For this review, take the finished solid that the model builds, in its own axes (mm). A direction names the side the tool comes from. Coordinates: 2 decimals unless noted, no trailing zeros. Loops run counter-clockwise (first coordinate to the right, second up) from the corner with the lowest first, then second, coordinate; pieces in that order, holes last. Notation, with made-up numbers: (47, 88) - (73, 88) arc R9 ccw to (73, 93) - close; hole circle Ø7 at (30.25, 54). An arc over 180 degrees is marked (long way). Use one line per item in the form item = value. Start each with the question number.
1. Machinability: for faces 1 (the face through (-0.33, -2.52, 3.76)), 2 (the face through (0, 0, -66.548)), which of the approach directions +Z, -Z, +X, -X, +Y, -Y give a long, thin tool a straight path to every point of the face, cutting with its end or side? Answer none if there is none.
2. For pin 1 Ø3 at (x, z) = (15.5, -5) entering from +Y; pin 2 Ø10 at (y, z) = (-14.5, -8.5) entering from +X; pin 3 Ø5 at (y, z) = (14.5, -31.5) entering from +X; pin 4 Ø22 at (x, y) = (5, 7) entering from +Z, all flat-tipped, find the tip position at first contact; note any pin that passes through.
3. Add section C-C on z = -31. Give the boundary of the cut face in (x, y) (3 decimals), and give its area (3 significant figures).
4. Add section A-A on y = 0. Give the boundary of the cut face in (x, z) (1 decimal).
5. To check wall thickness, follow probe 1 along Z at (x, y) = (0, 10.5); probe 2 along Y at (x, z) = (6.5, -52); probe 3 along Y at (x, z) = (-2.5, -26). State the ranges of each line that lie inside material, in increasing order.
Autodesk Inventor part; units mm, degrees
ref_plane "YZ Plane" through (0, 0, 0) normal (1, 0, 0) x (0, 1, 0)
ref_plane "XZ Plane" through (0, 0, 0) normal (0, 1, 0) x (-1, 0, 0)
ref_plane "XY Plane" through (0, 0, 0) normal (0, 0, 1) x (1, 0, 0)
sketch "Sketch1" plane through (0, 0, 0) normal (0, 0, 1) x (1, 0, 0)
  circle A0 centre (0, 0) radius 23.495
  circle A1 centre (0, 0) radius 2.54
  dimension "d0" = 46.99
  dimension "d3" = 5.08
extrude "Extrusion1" add sketch "Sketch1" against normal blind 66.548 contours A0 | A1
extrude "Extrusion2" add sketch "Sketch1" along normal blind 7.62 contours A1
fillet "Fillet1" radius 1.5875 1 edges at (-23.495, 0, 0)
fillet "Fillet2" radius 1.5875 1 edges at (-23.495, 0, -66.548)
properties part number "proxy 775 motor"
Conclusion:
q1.face_1 = +Z
q1.face_2 = -Z, +X, -X, +Y, -Y
q2.pin_1 = 18.87
q2.pin_2 = 21.49
q2.pin_3 = 20.2
q2.pin_4 = 7.62
q3.outline = circle Ø46.99 at (0, 0)
q3.area = 1,730 mm^2
q4.outline = (-23.5, -65) arc R1.6 ccw to (-21.9, -66.5) - (21.9, -66.5) arc R1.6 ccw to (23.5, -65) - (23.5, -1.6) arc R1.6 ccw to (21.9, 0) - (2.5, 0) - (2.5, 7.6) - (-2.5, 7.6) - (-2.5, 0) - (-21.9, 0) arc R1.6 ccw to (-23.5, -1.6) - close
q5.probe_1 = -66.55 to 0
q5.probe_2 = -22.58 to 22.58
q5.probe_3 = -23.36 to 23.36
